Autodesk Inventor part; units mm, degrees
ref_plane "YZ Plane" through (0, 0, 0) normal (1, 0, 0) x (0, 1, 0)
ref_plane "XZ Plane" through (0, 0, 0) normal (0, 1, 0) x (-1, 0, 0)
ref_plane "XY Plane" through (0, 0, 0) normal (0, 0, 1) x (1, 0, 0)
sketch "Boceto1" plane through (0, 0, 0) normal (0, 1, 0) x (-1, 0, 0)
  line L0 (0, 0) -> (0, -5)
  line L1 (0, -5) -> (13, -5)
  line L2 (13, -5) -> (13, 0)
  line L3 (13, 0) -> (0, 0)
  circle A0 centre (6.5, -2.5) radius 0.9
  dimension "d0" = 5
  dimension "d1" = 13
  dimension "d2" = 1.8
extrude "Extrusión1" add sketch "Boceto1" along normal blind 10.06
sketch "Boceto2" plane through (0, 10.06, 0) normal (0, 1, 0) x (1, 0, 0)
  circle A0 centre (-6.5, 2.5) radius 0.9
  point P0 (0, 0)
hole "Agujero1" at (-6.5, 10.06, -2.5) direction (0, -1, 0) diameter 4 depth 1.65
fillet "Empalme1" radius 1 4 edges at (0, 5.03, 0) (0, 5.03, -5) (-13, 5.03, 0) (-13, 5.03, -5)
properties part number "Soporte placa A1 - A2"
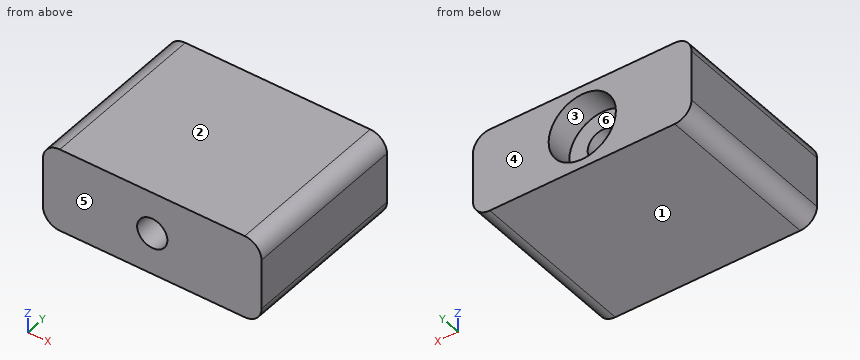
Could you check a few things on this model? Use its own coordinates, in mm. Face numbers are marked on the shaded views. A direction names the side the tool comes from. Round coordinates to 2 decimals unless told otherwise and drop trailing zeros. Order: outer loops, then holes, each group sorted by start corner. A loop starts at its lowest first (then second) coordinate and runs counter-clockwise, first axis right, second up. Notation, with made-up numbers: (88.5, 11.25) -> (106.5, 11.25) arc R30 cw to (106.5, 47.25) -> close; hole circle Ø11 at (78, 39). An arc over 180 degrees is marked (long way). One line per question, with ' | ' between items.
Q1. If I drill on line 1 (X direction, y = 5.5, z = -2.5); line 2 (Z direction, x = -6.5, y = 8.9); line 3 (X direction, y = 9, z = -2.5), over which ranges is the centre line in solid material (lowest first)? Write a range as from..to.
Computed values:
line 1: -13..-7.4, -5.6..0 | line 2: -5..-4.5, -0.5..0 | line 3: -13..-8.5, -4.5..0
Q2. We'd pull the mould along Z, two halves only. Please class the marked faces 1, 2, 3 and 4: released by +Z, released by -Z, zero draft, split by the parting line, or undercut.
Computed values:
face 1: released by -Z | face 2: released by +Z | face 3: undercut | face 4: zero draft
Q3. If we section it at B-B on x = -6.5: Write out the boundary of the cut face in (y, z), plus the area to 3 significant figures.
Computed values:
outline: (0, -5) -> (10.06, -5) -> (10.06, -4.5) -> (8.41, -4.5) -> (8.41, -3.4) -> (0, -3.4) -> close; (0, -1.6) -> (8.41, -1.6) -> (8.41, -0.5) -> (10.06, -0.5) -> (10.06, 0) -> (0, 0) -> close | area: 28.6 mm²
Q4. If we section it at A-A on y = 2.25: Write out the boundary of the cut face in (x, z), plus the area to 3 significant figures.
Computed values:
outline: (-13, -4) arc R1 ccw to (-12, -5) -> (-1, -5) arc R1 ccw to (0, -4) -> (0, -1) arc R1 ccw to (-1, 0) -> (-12, 0) arc R1 ccw to (-13, -1) -> close; hole circle Ø1.8 at (-6.5, -2.5) | area: 61.6 mm²
Q5. If we section it at D-D on z = -3.6: Write out the boundary of the cut face in (x, y), plus the area to 3 significant figures.
Computed values:
outline: (-13, 0) -> (0, 0) -> (0, 10.06) -> (-4.83, 10.06) -> (-4.83, 8.41) -> (-8.17, 8.41) -> (-8.17, 10.06) -> (-13, 10.06) -> close | area: 125 mm²
Q6. I'm going to push a flat-ended pin straight in: pin 1 (2.5 mm diameter, centred on x = -6.5, z = -2.5, fed in from +Y). Where does the tip first touch, or does it pass through?
Computed values:
pin 1: y = 8.41
Q7. Which directions (+Z, -Z, +X, -X, +Y, -Y) give clear straight access to the entire face, cutting with the end or side of a thin tool? Please do the marked faces 5 and 6.
Computed values:
face 5: +Z, -Z, +X, -X, -Y | face 6: +Y
Q8. If we section it at C-C on z = -2.5: Write out the boundary of the cut face in (x, y), plus the area to 3 significant figures.
Computed values:
outline: (-13, 0) -> (-7.4, 0) -> (-7.4, 8.41) -> (-8.5, 8.41) -> (-8.5, 10.06) -> (-13, 10.06) -> close; (-5.6, 0) -> (0, 0) -> (0, 10.06) -> (-4.5, 10.06) -> (-4.5, 8.41) -> (-5.6, 8.41) -> close | area: 109 mm²
